```python
from build123d import *

# Parameters (mm, degrees)
SKETCH1_R           = 3.175
BOSS_EXTRUDE1_DEPTH = 17.78
SKETCH2_R           = 3.96875
CUT_EXTRUDE1_DEPTH  = 33.3375
SKETCH3_R           = 4.7625
CUT_EXTRUDE2_DEPTH  = 4.7752


with BuildPart() as part:
    # Sketch1 → Boss-Extrude1 (new body)
    with BuildSketch(Plane.XY):
        with BuildLine():
            Line((0, 16.66875), (0, 7.62))
            ThreePointArc((0, 7.62), (7.62, 0), (0, -7.62))
            Line((0, -7.62), (0, -16.66875))
            Line((0, -16.66875), (-181.76875, -16.66875))
            Line((-181.76875, -16.66875), (-181.76875, -7.62))
            ThreePointArc((-181.76875, -7.62), (-189.38875, 0), (-181.76875, 7.62))
            Line((-181.76875, 7.62), (-181.76875, 16.66875))
            Line((-181.76875, 16.66875), (0, 16.66875))
        make_face()
        Circle(SKETCH1_R, mode=Mode.SUBTRACT)
        with Locations((-181.76875, 0)):
            Circle(SKETCH1_R, mode=Mode.SUBTRACT)
        with Locations((-90.884375, 0)):
            Circle(SKETCH1_R, mode=Mode.SUBTRACT)
    extrude(amount=-BOSS_EXTRUDE1_DEPTH)

    # Sketch2 → Cut-Extrude1 (cut)
    with BuildSketch(Plane(origin=(0, 16.66875, 0), x_dir=(1, 0, 0), z_dir=(0, 1, 0))):
        with Locations(Location((-12.7, 8.89, 0), (0, 0, 270))):
            Circle(SKETCH2_R)
        with Locations(Location((-63.5, 8.89, 0), (0, 0, 270))):
            Circle(SKETCH2_R)
        with Locations(Location((-114.3, 8.89, 0), (0, 0, 270))):
            Circle(SKETCH2_R)
        with Locations(Location((-165.1, 8.89, 0), (0, 0, 270))):
            Circle(SKETCH2_R)
    extrude(amount=-CUT_EXTRUDE1_DEPTH, mode=Mode.SUBTRACT)

    # Sketch3 → Cut-Extrude2 (cut)
    with BuildSketch(Plane.XY):
        Circle(SKETCH3_R)
        with Locations((-90.884375, 0)):
            Circle(SKETCH3_R)
        with Locations((-181.76875, 0)):
            Circle(SKETCH3_R)
    extrude(amount=-CUT_EXTRUDE2_DEPTH, mode=Mode.SUBTRACT)


solid = part.part
```
Model file for the job. Use its own axes, mm. A direction names the side the tool comes from. Coordinates: 2 decimals unless noted, no trailing zeros. Order: outer loops, then holes, each group sorted by start corner. A loop starts at its lowest first (then second) coordinate and runs counter-clockwise, first axis right, second up. Notation, with made-up numbers: (1, 65) - (52, 65) arc R32 ccw to (52, 101) - close; hole circle Ø4 at (-16, 66). An arc over 180 degrees is marked (long way). Return JSON: item names as keys, results as strings. Group by question number.
1) Saw through at C-C, the plane y = -14. Write the cut outline in (x, z), plus the area to 3 significant figures.
2) Tool access for faces 1 (the flat face through (-181.769, 12, -9)), 2 (the flat face through (0, 12, -9)), 3 (the flat face through (0, -12, -9)), 4 (the flat face through (-181.769, -12, -9)): list every direction of +Z, -Z, +X, -X, +Y, -Y with a clear straight run to the whole face (end or side of a thin tool).
3) Flat gauge pins, fed straight in: P1, Ø4.5, axis at y = 13, z = -12.5, coming from the +X side; P2, Ø5, axis at y = -3.5, z = -8, coming from the +X side; P3, Ø10, axis at y = -14, z = -8, coming from the -X side. Where does each tip first touch, or does it go through?
4) Mould opens along Y. For faces 5 (the cylindrical face through (7.62, 0.17, -8.77)), 6 (the cylindrical face through (-16.22, 0.23, -7.06)), 7 (the cylindrical face through (-0.69, -3.1, -11.19)) say: released by +Y, released by -Y, zero draft, split by the parting line, or undercut.
5) Saw through at A-A, the plane z = -8.89. Write the cut outline in (x, y) (3 decimals).
6) Probe line 1 (X direction, y = 8, z = -8.89); line 2 (Y direction, x = -90.5, z = -11.75); line 3 (X direction, y = 4, z = -9). List the from-to ranges inside material, lowest first. Write a range as from..to.
7) Saw through at B-B, the plane x = -63.5. Write the cut outline in (y, z), plus the area to 3 significant figures.
Values found:
{
 "1": {"outline": "(-181.77, -17.78) - (0, -17.78) - (0, 0) - (-181.77, 0) - close; hole circle Ø7.94 at (-165.1, -8.89); hole circle Ø7.94 at (-114.3, -8.89); hole circle Ø7.94 at (-63.5, -8.89); hole circle Ø7.94 at (-12.7, -8.89)", "area": "3,030 mm²"},
 "2": {"face 1": "+Z, -Z, -X, +Y", "face 2": "+Z, -Z, +X, +Y", "face 3": "+Z, -Z, +X, -Y", "face 4": "+Z, -Z, -X, -Y"},
 "3": {"P1": "stops at x = 0", "P2": "stops at x = 7.55", "P3": "stops at x = -181.77"},
 "4": {"face 5": "split by the parting line", "face 6": "zero draft", "face 7": "undercut"},
 "5": {"outline": "(-181.769, -16.669) - (-169.069, -16.669) - (-169.069, 16.669) - (-181.769, 16.669) - (-181.769, 7.62) arc R7.62 ccw to (-181.769, -7.62) - close; (-161.131, -16.669) - (-118.269, -16.669) - (-118.269, 16.669) - (-161.131, 16.669) - close; (-110.331, -16.669) - (-67.469, -16.669) - (-67.469, 16.669) - (-110.331, 16.669) - close; (-59.531, -16.669) - (-16.669, -16.669) - (-16.669, 16.669) - (-59.531, 16.669) - close; (-8.731, -16.669) - (0, -16.669) - (0, -7.62) arc R7.62 ccw to (0, 7.62) - (0, 16.669) - (-8.731, 16.669) - close; hole circle Ø6.35 at (-181.769, 0); hole circle Ø6.35 at (-90.884, 0); hole circle Ø6.35 at (0, 0)"},
 "6": {"line 1": "x = -181.77..-169.07, -161.13..-118.27, -110.33..-67.47, -59.53..-16.67, -8.73..0", "line 2": "y = -16.67..-3.15, 3.15..16.67", "line 3": "x = -188.25..-169.07, -161.13..-118.27, -110.33..-67.47, -59.53..-16.67, -8.73..6.49"},
 "7": {"outline": "(-16.67, -17.78) - (16.67, -17.78) - (16.67, -12.86) - (-16.67, -12.86) - close; (-16.67, -4.92) - (16.67, -4.92) - (16.67, 0) - (-16.67, 0) - close", "area": "328 mm²"}
}
